from build123d import *

# Parameters (mm, degrees)
SKETCH1_W                        = 118.56
SKETCH1_H                        = 42
BOSS_EXTRUDE1_DEPTH              = 41.5
SKETCH2_W                        = 107.56
SKETCH2_H                        = 36
CUT_EXTRUDE1_DEPTH               = 37.5
FILLET1_R                        = 4
CUT_EXTRUDE2_REACH               = 120.56
SKETCH3_R                        = 15.5
CUT_EXTRUDE5_REACH               = 44
SKETCH22_W                       = 8
SKETCH22_H                       = 42
BOSS_EXTRUDE3_DEPTH              = 11
SKETCH23_W                       = 8
SKETCH23_H                       = 42
BOSS_EXTRUDE4_DEPTH              = 11
F_4_0MM_DOWEL_HOLE2_D            = 4
F_4_0MM_DOWEL_HOLE2_DEPTH        = 4.5
F_4_0MM_DOWEL_HOLE2_TIP          = 1.201721238
CBORE_FOR_M5_SHCS1_D             = 5.3
CBORE_FOR_M5_SHCS1_CBORE_D       = 10
CBORE_FOR_M5_SHCS1_CBORE_DEPTH   = 5
F_5_0MM_DOWEL_HOLE1_D            = 5
F_5_0MM_DOWEL_HOLE1_DEPTH        = 3
F_5_0MM_DOWEL_HOLE2_D            = 5
F_5_0MM_DOWEL_HOLE2_DEPTH        = 3
M3X0_5_TAPPED_HOLE1_D            = 2.5
M3X0_5_TAPPED_HOLE1_DEPTH        = 3
M3X0_5_TAPPED_HOLE2_D            = 2.5
M3X0_5_TAPPED_HOLE2_DEPTH        = 3
F_3_0MM_DOWEL_HOLE1_D            = 3
F_3_0MM_DOWEL_HOLE1_DEPTH        = 3
F_3_0MM_DOWEL_HOLE1_TIP          = 0.901290929
CBORE_FOR_M2_5_SHCS1_D           = 2.9
CBORE_FOR_M2_5_SHCS1_DEPTH       = 4
CBORE_FOR_M2_5_SHCS1_CBORE_D     = 5.5
CBORE_FOR_M2_5_SHCS1_CBORE_DEPTH = 2.5
F_1_16_0_0625_DOWEL_HOLE1_D      = 1.5875
F_1_16_0_0625_DOWEL_HOLE1_DEPTH  = 3
F_1_16_0_0625_DOWEL_HOLE1_TIP    = 0.476933116
CBORE_FOR_M2_SHCS1_D             = 2.2
CBORE_FOR_M2_SHCS1_DEPTH         = 4
CBORE_FOR_M2_SHCS1_CBORE_D       = 4.4
CBORE_FOR_M2_SHCS1_CBORE_DEPTH   = 2
F_3_0MM_DOWEL_HOLE2_D            = 3
F_3_0MM_DOWEL_HOLE2_DEPTH        = 3
F_3_0MM_DOWEL_HOLE2_TIP          = 0.901290929
CBORE_FOR_M2_5_SHCS2_D           = 2.9
CBORE_FOR_M2_5_SHCS2_DEPTH       = 4
CBORE_FOR_M2_5_SHCS2_CBORE_D     = 5.5
CBORE_FOR_M2_5_SHCS2_CBORE_DEPTH = 2.5
M2X0_4_TAPPED_HOLE1_D            = 1.6
M2X0_4_TAPPED_HOLE1_DEPTH        = 5.2
M2X0_4_TAPPED_HOLE1_TIP          = 0.480688495


with BuildPart() as part:
    # Sketch1 → Boss-Extrude1 (new body)
    with BuildSketch(Plane(origin=(0, 0, 0), x_dir=(1, 0, 0), z_dir=(0, 1, 0))):
        Rectangle(SKETCH1_W, SKETCH1_H)
    extrude(amount=BOSS_EXTRUDE1_DEPTH)

    # Sketch2 → Cut-Extrude1 (cut)
    with BuildSketch(Plane(origin=(0, 41.5, 0), x_dir=(1, 0, 0), z_dir=(0, 1, 0))):
        with Locations((2.5, 0)):
            Rectangle(SKETCH2_W, SKETCH2_H)
    extrude(amount=-CUT_EXTRUDE1_DEPTH, mode=Mode.SUBTRACT)

    # Fillet1
    fillet1_edges = [part.edges().sort_by_distance(p)[0] for p in [
        (-51.28, 22.75, 18),
        (-51.28, 22.75, -18),
        (56.28, 22.75, -18),
        (56.28, 22.75, 18),
    ]]
    fillet(fillet1_edges, radius=FILLET1_R)

    # Sketch3 → Cut-Extrude2 (cut, up to next)
    with BuildSketch(Plane.ZY.offset(59.28), mode=Mode.PRIVATE) as cut_extrude2_sk1:
        with Locations((0, 20.5)):
            Circle(SKETCH3_R)
    cut_extrude2_tool1 = extrude(cut_extrude2_sk1.sketch, amount=-CUT_EXTRUDE2_REACH, mode=Mode.PRIVATE) & part.part
    add(cut_extrude2_tool1.solids().sort_by_distance((-59.28, 20.5, 0))[0], mode=Mode.SUBTRACT)

    # Sketch10 → Cut-Extrude5 (cut, up to next)
    with BuildSketch(Plane.XY.offset(21), mode=Mode.PRIVATE) as cut_extrude5_sk1:
        with BuildLine():
            Line((26.08, 32.25), (26.08, 8.75))
            ThreePointArc((26.08, 8.75), (24.18, 6.85), (22.28, 8.75))
            Line((22.28, 8.75), (22.28, 32.25))
            ThreePointArc((22.28, 32.25), (24.18, 34.15), (26.08, 32.25))
        make_face()
    cut_extrude5_tool1 = extrude(cut_extrude5_sk1.sketch, amount=-CUT_EXTRUDE5_REACH, mode=Mode.PRIVATE) & part.part
    add(cut_extrude5_tool1.solids().sort_by_distance((24.18, 20.5, 21))[0], mode=Mode.SUBTRACT)

    # Sketch22 → Boss-Extrude3 (add)
    with BuildSketch(Plane.XZ):
        with Locations((-55.28, 0)):
            Rectangle(SKETCH22_W, SKETCH22_H)
    extrude(amount=BOSS_EXTRUDE3_DEPTH)

    # Sketch23 → Boss-Extrude4 (add)
    with BuildSketch(Plane(origin=(0, 41.5, 0), x_dir=(1, 0, 0), z_dir=(0, 1, 0))):
        with Locations((-55.28, 0)):
            Rectangle(SKETCH23_W, SKETCH23_H)
    extrude(amount=BOSS_EXTRUDE4_DEPTH)

    # Ø4.0mm Dowel Hole2
    with Locations(Plane.ZY.offset(59.28)):
        with Locations((0, 46.75), (0, -5.75)):
            Hole(F_4_0MM_DOWEL_HOLE2_D / 2, depth=F_4_0MM_DOWEL_HOLE2_DEPTH)
            with Locations((0, 0, -(F_4_0MM_DOWEL_HOLE2_DEPTH + F_4_0MM_DOWEL_HOLE2_TIP / 2))):  # 118° drill point
                Cone(0, F_4_0MM_DOWEL_HOLE2_D / 2, F_4_0MM_DOWEL_HOLE2_TIP, mode=Mode.SUBTRACT)

    # CBORE for M5 SHCS1 (through all)
    with Locations(Plane(origin=(-51.28, 0, 0), x_dir=(0, 0, -1), z_dir=(1, 0, 0))):
        with Locations((-15, 46.75), (15, 46.75), (-15, -5.75), (15, -5.75)):
            CounterBoreHole(CBORE_FOR_M5_SHCS1_D / 2, CBORE_FOR_M5_SHCS1_CBORE_D / 2, CBORE_FOR_M5_SHCS1_CBORE_DEPTH)

    # Ø5.0mm Dowel Hole1
    with Locations(Plane(origin=(0, 0, -21), x_dir=(-1, 0, 0), z_dir=(0, 0, -1))):
        with Locations((-2.721503605, 20.5), (-37.207540509, 20.5)):
            Hole(F_5_0MM_DOWEL_HOLE1_D / 2, depth=F_5_0MM_DOWEL_HOLE1_DEPTH)

    # Ø5.0mm Dowel Hole2
    with Locations(Plane(origin=(59.28, 0, 0), x_dir=(0, 0, -1), z_dir=(1, 0, 0))):
        with Locations((0, 20.5)):
            Hole(F_5_0MM_DOWEL_HOLE2_D / 2, depth=F_5_0MM_DOWEL_HOLE2_DEPTH)

    # M3x0.5 Tapped Hole1
    with Locations(Plane(origin=(0, 0, -21), x_dir=(-1, 0, 0), z_dir=(0, 0, -1))):
        with Locations((9.778496395, 8), (-15.221503605, 8), (-15.221503605, 33), (9.778496395, 33), (-24.656395143, 7.948854634), (-49.758685875, 7.948854634), (-49.758685875, 33.051145366), (-24.656395143, 33.051145366)):
            Hole(M3X0_5_TAPPED_HOLE1_D / 2, depth=M3X0_5_TAPPED_HOLE1_DEPTH)

    # M3x0.5 Tapped Hole2
    with Locations(Plane(origin=(59.28, 0, 0), x_dir=(0, 0, -1), z_dir=(1, 0, 0))):
        with Locations((12.5, 8), (-12.798632739, 8), (-12.5, 33), (12.5, 33)):
            Hole(M3X0_5_TAPPED_HOLE2_D / 2, depth=M3X0_5_TAPPED_HOLE2_DEPTH)

    # Ø3.0mm Dowel Hole1
    with Locations(Plane(origin=(0, 4, 0), x_dir=(1, 0, 0), z_dir=(0, 1, 0))):
        with Locations((-4.703117598, -10.253048327), (12.974551932, 7.424621202)):
            Hole(F_3_0MM_DOWEL_HOLE1_D / 2, depth=F_3_0MM_DOWEL_HOLE1_DEPTH)
            with Locations((0, 0, -(F_3_0MM_DOWEL_HOLE1_DEPTH + F_3_0MM_DOWEL_HOLE1_TIP / 2))):  # 118° drill point
                Cone(0, F_3_0MM_DOWEL_HOLE1_D / 2, F_3_0MM_DOWEL_HOLE1_TIP, mode=Mode.SUBTRACT)

    # CBORE for M2.5 SHCS1
    with Locations(Plane(origin=(0, 0, 0), x_dir=(-1, 0, 0), z_dir=(0, -1, 0))):
        with Locations((-4.170075035, -1.448571431)):
            CounterBoreHole(CBORE_FOR_M2_5_SHCS1_D / 2, CBORE_FOR_M2_5_SHCS1_CBORE_D / 2, CBORE_FOR_M2_5_SHCS1_CBORE_DEPTH, depth=CBORE_FOR_M2_5_SHCS1_DEPTH)

    # 1/16 (0.0625) Dowel Hole1
    with Locations(Plane(origin=(0, 4, 0), x_dir=(1, 0, 0), z_dir=(0, 1, 0))):
        with Locations((41.086220165, -3.878679656), (33.328860853, 3.878679656)):
            Hole(F_1_16_0_0625_DOWEL_HOLE1_D / 2, depth=F_1_16_0_0625_DOWEL_HOLE1_DEPTH)
            with Locations((0, 0, -(F_1_16_0_0625_DOWEL_HOLE1_DEPTH + F_1_16_0_0625_DOWEL_HOLE1_TIP / 2))):  # 118° drill point
                Cone(0, F_1_16_0_0625_DOWEL_HOLE1_D / 2, F_1_16_0_0625_DOWEL_HOLE1_TIP, mode=Mode.SUBTRACT)

    # CBORE for M2 SHCS1
    with Locations(Plane(origin=(0, 0, 0), x_dir=(-1, 0, 0), z_dir=(0, -1, 0))):
        with Locations((-41.086220165, 3.878679656), (-33.328860853, -3.878679656)):
            CounterBoreHole(CBORE_FOR_M2_SHCS1_D / 2, CBORE_FOR_M2_SHCS1_CBORE_D / 2, CBORE_FOR_M2_SHCS1_CBORE_DEPTH, depth=CBORE_FOR_M2_SHCS1_DEPTH)

    # Ø3.0mm Dowel Hole2
    with Locations(Plane(origin=(0, 4, 0), x_dir=(1, 0, 0), z_dir=(0, 1, 0))):
        with Locations((23.894423104, -11.836644244), (23.126634177, 10.14995395)):
            Hole(F_3_0MM_DOWEL_HOLE2_D / 2, depth=F_3_0MM_DOWEL_HOLE2_DEPTH)
            with Locations((0, 0, -(F_3_0MM_DOWEL_HOLE2_DEPTH + F_3_0MM_DOWEL_HOLE2_TIP / 2))):  # 118° drill point
                Cone(0, F_3_0MM_DOWEL_HOLE2_D / 2, F_3_0MM_DOWEL_HOLE2_TIP, mode=Mode.SUBTRACT)

    # CBORE for M2.5 SHCS2
    with Locations(Plane(origin=(0, 0, 0), x_dir=(-1, 0, 0), z_dir=(0, -1, 0))):
        with Locations((-23.458179395, 0.655741094)):
            CounterBoreHole(CBORE_FOR_M2_5_SHCS2_D / 2, CBORE_FOR_M2_5_SHCS2_CBORE_D / 2, CBORE_FOR_M2_5_SHCS2_CBORE_DEPTH, depth=CBORE_FOR_M2_5_SHCS2_DEPTH)

    # M2x0.4 Tapped Hole1
    with Locations(Plane(origin=(0, 41.5, 0), x_dir=(1, 0, 0), z_dir=(0, 1, 0))):
        with Locations((57.28, -19.5), (3.420478131, -19.5), (-48.78, -19.5), (-48.78, 19.5), (3.420478131, 19.5), (57.28, 19.5)):
            Hole(M2X0_4_TAPPED_HOLE1_D / 2, depth=M2X0_4_TAPPED_HOLE1_DEPTH)
            with Locations((0, 0, -(M2X0_4_TAPPED_HOLE1_DEPTH + M2X0_4_TAPPED_HOLE1_TIP / 2))):  # 118° drill point
                Cone(0, M2X0_4_TAPPED_HOLE1_D / 2, M2X0_4_TAPPED_HOLE1_TIP, mode=Mode.SUBTRACT)


solid = part.part
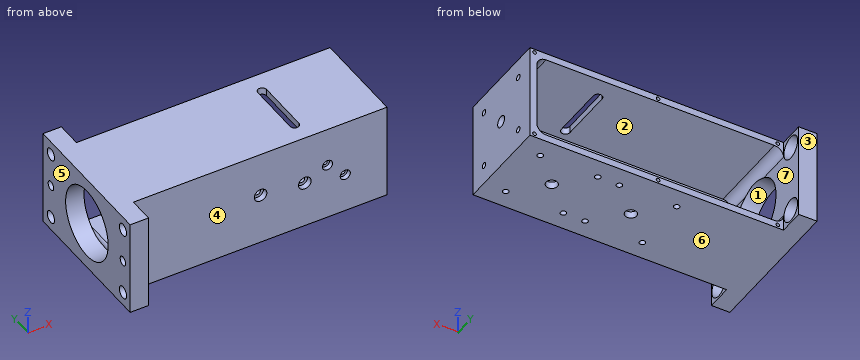
Could you check a few things on this model? Use its own coordinates, in mm. Face numbers are marked on the shaded views. A direction names the side the tool comes from. Give positions to 0.01 mm unless a question says otherwise; leave off trailing zeros. Write each loop counter-clockwise with the first axis right and the second up, starting at its lowest first coordinate (ties: lowest second). Pieces come first, ordered by that corner, then holes. Notation, with made-up numbers: (37, -33) -> (64, -33) arc R6 ccw to (64, -25) -> close; hole circle Ø5 at (2.25, -25). An arc over 180 degrees is marked (long way). Answer as CSV lines item,"result". Start each with the question number.
(1) If we mould it in two halves opening along Z, with no side actions, what happens to the marked faces 5, 6 and 7? For each: +Z half, -Z half, draft (parallel to the pull), parting line (faces both ways), or undercut.
(2) Please list where these lines run through material, in increasing order: line 1 (X direction, y = 38.9, z = 19.5); line 2 (X direction, y = 13, z = 14); line 3 (Z direction, x = -25.5, y = 34.5).
(3) If we section it at C-C, the plane x = 44.5: Write out the boundary of the cut face in (y, z).
(4) If we section it at A-A, the plane y = 20.5: Give the number of separate pieces and of enclosed holes in the cut face, and give its area (3 significant figures).
(5) If we section it at B-B, the plane y = 37.5: Write out the boundary of the cut face in (x, z), and give its area (3 significant figures).
(6) Which directions (+Z, -Z, +X, -X, +Y, -Y) give clear straight access to the entire face, cutting with the end or side of a thin tool? Please do the marked faces 1, 2, 3 and 4.
(7) I'm going to push flat-ended pins straight in: pin 1 Ø4 at (x, z) = (-14, 12.5) entering from +Y; pin 2 Ø12 at (x, z) = (-25.5, -1) entering from -Y; pin 3 Ø2.5 at (y, z) = (-5.75, 0) entering from -X. Where does each tip first touch, or does it pass through?
Answer list:
1,face 5,"draft"
1,face 6,"-Z half"
1,face 7,"undercut"
2,line 1,"-59.28 to -49.58, -47.98 to 2.62, 4.22 to 56.48, 58.08 to 59.28"
2,line 2,"-59.28 to -51.28, 56.28 to 59.28"
2,line 3,"-21 to -18, 18 to 21"
3,outline,"(0, -21) -> (41.5, -21) -> (41.5, -18) -> (4, -18) -> (4, 18) -> (41.5, 18) -> (41.5, 21) -> (0, 21) -> close"
4,separate pieces,"5"
4,enclosed holes,"0"
4,area,"816 mm^2"
5,outline,"(-59.28, -21) -> (59.28, -21) -> (59.28, 21) -> (-59.28, 21) -> close; hole (-51.28, -14) arc R4 ccw to (-47.28, -18) -> (52.28, -18) arc R4 ccw to (56.28, -14) -> (56.28, 14) arc R4 ccw to (52.28, 18) -> (-47.28, 18) arc R4 ccw to (-51.28, 14) -> close; hole circle Ø1.6 at (-48.78, -19.5); hole circle Ø1.6 at (-48.78, 19.5); hole circle Ø1.6 at (3.42, -19.5); hole circle Ø1.6 at (3.42, 19.5); hole circle Ø1.6 at (57.28, -19.5); hole circle Ø1.6 at (57.28, 19.5)"
5,area,"1,110 mm^2"
6,face 1,"-X"
6,face 2,"+Y"
6,face 3,"+Z, -Z, +X, -X, +Y"
6,face 4,"+Z, -Z, +X, -Y"
7,pin 1,"y = 4"
7,pin 2,"y = 0"
7,pin 3,"x = -54.33"
